Can you work these out from the model? Positions are in its coordinate system, mm. Face numbers are marked on the shaded views. A direction names the side the tool comes from. Round coordinates to 2 decimals unless told otherwise and drop trailing zeros. Order: outer loops, then holes, each group sorted by start corner. A loop starts at its lowest first (then second) coordinate and runs counter-clockwise, first axis right, second up.
Q1. If we section it at C-C (y = 18.5): Please give me the cut outline in (x, z).
Q2. If I drill on line 1 (X direction, y = 14.5, z = 12.75); line 2 (Y direction, x = 15, z = 24.75); line 3 (X direction, y = 16.25, z = 11), over which ranges is the centre line in solid material (lowest first)?
Q3. If we section it at D-D (x = 0): Please give me the cut outline in (y, z).
Q4. For the marked faces 5, 6, 7, 8 and 9, which set-ups out of +Z, -Z, +X, -X, +Y, -Y let a thin tool reach every point of the face, with its end or its side?
Q5. Will these pins go through, and if not, where does the flat tip stop? P1, Ø2, axis at x = -16, y = 8.5, coming from the +Z side; P2, Ø6, axis at x = -15, y = 10, coming from the -Z side; P3, Ø3, axis at y = 7, z = 14.5, coming from the -X side.
Q6. We'd pull the mould along X, two halves only. Please class the marked faces 1, 2, 3 and 4: pulls with the +X half, pulls with the -X half, needs draft (parallel to the pull), parting line crosses it, or undercut.
Q7. If we section it at B-B (x = -15): Please give me the cut outline in (y, z), plus the area to 4 significant figures.
Q8. If we section it at A-A (z = 3.5): Please give me the cut outline in (x, y).
Autodesk Inventor part; units mm, degrees
ref_plane "YZ Plane" through (0, 0, 0) normal (1, 0, 0) x (0, 1, 0)
ref_plane "XZ Plane" through (0, 0, 0) normal (0, 1, 0) x (-1, 0, 0)
ref_plane "XY Plane" through (0, 0, 0) normal (0, 0, 1) x (1, 0, 0)
sketch "Szkic1" plane through (0, 0, 0) normal (0, 1, 0) x (-1, 0, 0)
  line L0 (25, 20) -> (5, 20)
  line L1 (5, 20) -> (5, 0)
  line L2 (5, 0) -> (25, 0)
  line L3 (25, 0) -> (25, 20)
  line L4 (-5, 20) -> (-25, 20)
  line L5 (-25, 20) -> (-25, 0)
  line L6 (-25, 0) -> (-5, 0)
  line L7 (-5, 0) -> (-5, 20)
  line L8 (25, 0) -> (-25, 0)
  line L9 (-25, 0) -> (-25, 30)
  line L10 (-25, 30) -> (25, 30)
  line L11 (25, 30) -> (25, 0)
  line L12 (-25, 30) -> (-35, 30)
  line L13 (-35, 30) -> (-35, 0)
  line L14 (-35, 0) -> (-25, 0)
  line L15 (-25, 0) -> (-25, 30)
  line L16 (-25, 12.5) -> (-24, 12.5)
  line L17 (-23, 11.5) -> (-23, 8.5)
  line L18 (-24, 7.5) -> (-25, 7.5)
  line L19 (-25, 7.5) -> (-25, 12.5)
  arc A0 (-23, 11.5) -> (-24, 12.5) centre (-24, 11.5) ccw
  arc A1 (-24, 7.5) -> (-23, 8.5) centre (-24, 8.5) ccw
  point P0 (0, 0)
  point P1 (-15, 20)
  point P2 (15, 20)
  point P3 (15, 0)
  point P4 (-5, 0)
  point P5 (5, 0)
  point P6 (-23, 7.5)
  point P7 (-23, 12.5)
  dimension "d0" = 20
  dimension "d1" = 20
  dimension "d2" = 20
  dimension "d3" = 20
  dimension "d4" = 50
  dimension "d5" = 25
  dimension "d6" = 10
  dimension "d28" = 10
  dimension "d29" = 5
  dimension "d30" = 7.5
  dimension "d31" = 2
  dimension "d33" = 1
extrude "Wyciągnięcie proste1" add sketch "Szkic1" along normal blind 20 contours L0 L1 L8 L7 L4 L9 L10 L11 | L9 L5 L14 L13 L12 | L16 A0 L17 A1 L18 L5
sketch "Szkic2" plane through (5, 0, 0) normal (0, 0, -1) x (-1, 0, 0)
  circle A0 centre (5, 10) radius 3.25
  circle A1 centre (20, 10) radius 2.25
  circle A2 centre (-10, 10) radius 2.25
  line L0 (0, 0) -> (0, 20)
  line L1 (0, 0) -> (10, 0)
  line L2 (-20, 0) -> (0, 0)
  line L3 (30, 0) -> (30, 20)
  circle A3 centre (-10, 10) radius 4
  circle A4 centre (20, 10) radius 4
  line L4 (1.8246, 15.5) -> (8.1754, 15.5)
  line L5 (8.1754, 15.5) -> (11.3509, 10)
  line L6 (11.3509, 10) -> (8.1754, 4.5)
  line L7 (8.1754, 4.5) -> (1.8246, 4.5)
  line L8 (1.8246, 4.5) -> (-1.3509, 10)
  line L9 (-1.3509, 10) -> (1.8246, 15.5)
  line L10 (-20, 0) -> (-20, 20)
  point P0 (5, 0)
  dimension "d9" = 6.5
  dimension "d10" = 5
  dimension "d11" = 10
  dimension "d13" = 10
  dimension "d14" = 10
  dimension "d15" = 4.5
  dimension "d16" = 4.5
  dimension "d20" = 8
  dimension "d21" = 8
  dimension "d25" = 11
  dimension "d32" = 10
extrude "Wyciągnięcie proste2" cut sketch "Szkic2" against normal through all contours A0 | A1 | A2
extrude "Wyciągnięcie proste3" cut sketch "Szkic2" along normal blind 5 from surface at -30 contours A0 | L8 L9 L0 | L0 L9 L4 L5 L6 L7 L8
fillet "Zaokrąglenie1" radius 6 2 edges at (-25, 10, 30) (35, 10, 30)
extrude "Wyciągnięcie proste4" cut sketch "Szkic2" along normal blind 1 from surface at -30 contours A1 | A2 | A3 | A4
properties part number "ZItemMountCable" material "Tworzywo sztuczne ABS"
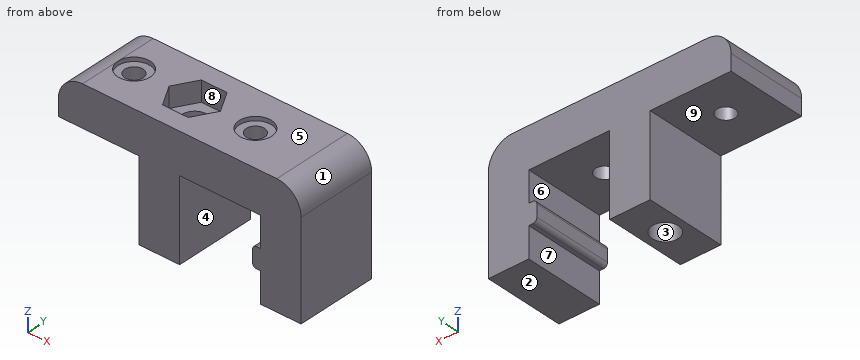
Solution:
1. outline: (-25, 20) - (-5, 20) - (-5, 0) - (5, 0) - (5, 20) - (25, 20) - (25, 12.5) - (24, 12.5) arc R1 ccw to (23, 11.5) - (23, 8.5) arc R1 ccw to (24, 7.5) - (25, 7.5) - (25, 0) - (35, 0) - (35, 24) arc R6 ccw to (29, 30) - (-19, 30) arc R6 ccw to (-25, 24) - close
2. line 1: x = -5 to 5, 25 to 35
2. line 2: y = 0 to 7.75, 12.25 to 20
2. line 3: x = -5 to 5, 23 to 35
3. outline: (0, 0) - (6.75, 0) - (6.75, 25) - (4.5, 25) - (4.5, 30) - (0, 30) - close; (13.25, 0) - (20, 0) - (20, 30) - (15.5, 30) - (15.5, 25) - (13.25, 25) - close
4. face 5: +Z, +X, -X, +Y, -Y
4. face 6: +Y, -Y
4. face 7: -Z, +Y, -Y
4. face 8: +Z
4. face 9: -Z, -X, +Y, -Y
5. P1: stops at z = 29
5. P2: stops at z = 20
5. P3: stops at x = -5
6. face 1: pulls with the +X half
6. face 2: needs draft
6. face 3: undercut
6. face 4: undercut
7. outline: (0, 20) - (7.75, 20) - (7.75, 29) - (6, 29) - (6, 30) - (0, 30) - close; (12.25, 20) - (20, 20) - (20, 30) - (14, 30) - (14, 29) - (12.25, 29) - close
7. area: 151.5 mm2
8. outline: (-5, 0) - (5, 0) - (5, 20) - (-5, 20) - close; (25, 0) - (35, 0) - (35, 20) - (25, 20) - close; hole circle Ø6.5 at (0, 10)
